from build123d import *

# Parameters (mm, degrees)
ESBO_O1_W                = 51.12
ESBO_O1_H                = 44.13
ESBO_O1_R                = 2
RESSALTO_EXTRUS_O1_DEPTH = 3


with BuildPart() as part:
    # Esboço1 → Ressalto-extrusão1 (new body)
    with BuildSketch(Plane(origin=(0, 0, 0), x_dir=(1, 0, 0), z_dir=(0, 1, 0))):
        with Locations((11.56, 12.065)):
            Rectangle(ESBO_O1_W, ESBO_O1_H)
        with Locations(Location((31.12, 12.065, 0), (0, 0, 270))):
            Circle(ESBO_O1_R, mode=Mode.SUBTRACT)
        with Locations(Location((-8, 12.065, 0), (0, 0, 270))):
            Circle(ESBO_O1_R, mode=Mode.SUBTRACT)
        with Locations(Location((11.56, 28.13, 0), (0, 0, 270))):
            Circle(ESBO_O1_R, mode=Mode.SUBTRACT)
        with Locations(Location((11.56, -4, 0), (0, 0, 270))):
            Circle(ESBO_O1_R, mode=Mode.SUBTRACT)
        Polygon((23.12, 24.13), (23.12, 18.13), (27.12, 18.13), (27.12, 6), (23.12, 6), (23.12, 0), (0, 0), (0, 6), (-4, 6), (-4, 18.13), (0, 18.13), (0, 24.13), align=None, mode=Mode.SUBTRACT)
    extrude(amount=RESSALTO_EXTRUS_O1_DEPTH)


solid = part.part
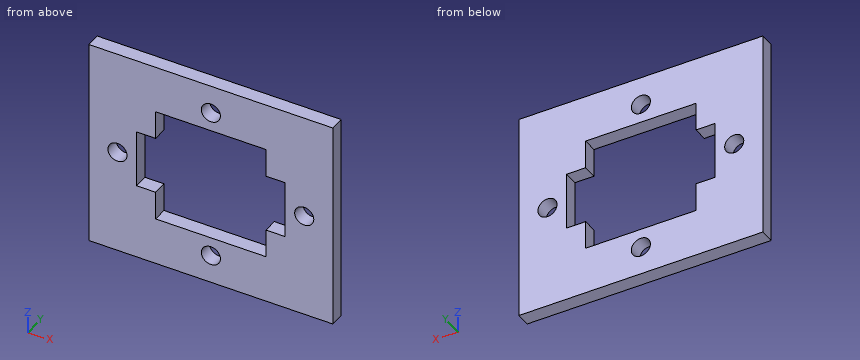
Here's how the part is built. I have some questions about the finished solid (model axes, mm). Coordinates: 2 decimals unless noted, no trailing zeros. Order: outer loops, then holes, each group sorted by start corner. A loop starts at its lowest first (then second) coordinate and runs counter-clockwise, first axis right, second up. Notation, with made-up numbers: (34.25, 29.25) -> (52.25, 29.25) arc R22 ccw to (52.25, 63.25) -> close; hole circle Ø11 at (-7, -2.5). An arc over 180 degrees is marked (long way). Answer in a Markdown table with one row per item.
(1) I want a section at D-D on x = 17.5. List the corners of the cut face in (y, z) for me, then the cut area to 3 significant figures.
Answer key:
| item | result |
|---|---|
| outline | (0, -34.13) -> (3, -34.13) -> (3, -24.13) -> (0, -24.13) -> close; (0, 0) -> (3, 0) -> (3, 10) -> (0, 10) -> close |
| area | 60.0 mm^2 |
(2) I want a section at B-B on z = 4. List the corners of the cut face in (x, y) for me, then the cut area to 3 significant figures.
Answer key:
| item | result |
|---|---|
| outline | (-14, 0) -> (9.56, 0) -> (9.56, 3) -> (-14, 3) -> close; (13.56, 0) -> (37.12, 0) -> (37.12, 3) -> (13.56, 3) -> close |
| area | 141 mm^2 |
(3) Will this pin go through, and if not, where does the flat tip stop? pin 1 Ø12 at (x, z) = (11.5, -23) entering from +Y.
Answer key:
| item | result |
|---|---|
| pin 1 | y = 3 |
(4) Please list where these lines run through material, in increasing order: probe 1 along Z at (x, y) = (25.5, 1.3); probe 2 along Z at (x, y) = (14.5, 0.8); probe 3 along X at (y, z) = (0.85, -18).
Answer key:
| item | result |
|---|---|
| probe 1 | -34.13 to -18.13, -6 to 10 |
| probe 2 | -34.13 to -24.13, 0 to 10 |
| probe 3 | -14 to -4, 27.12 to 37.12 |
(5) I want a section at A-A on x = 11.56. List the corners of the cut face in (y, z) for me, then the cut area to 3 significant figures.
Answer key:
| item | result |
|---|---|
| outline | (0, -34.13) -> (3, -34.13) -> (3, -30.13) -> (0, -30.13) -> close; (0, -26.13) -> (3, -26.13) -> (3, -24.13) -> (0, -24.13) -> close; (0, 0) -> (3, 0) -> (3, 2) -> (0, 2) -> close; (0, 6) -> (3, 6) -> (3, 10) -> (0, 10) -> close |
| area | 36.0 mm^2 |
(6) I want a section at C-C on y = 1.4. List the corners of the cut face in (x, z) for me (3 decimals).
Answer key:
| item | result |
|---|---|
| outline | (-14, -34.13) -> (37.12, -34.13) -> (37.12, 10) -> (-14, 10) -> close; hole circle Ø4 at (-8, -12.065); hole (-4, -18.13) -> (0, -18.13) -> (0, -24.13) -> (23.12, -24.13) -> (23.12, -18.13) -> (27.12, -18.13) -> (27.12, -6) -> (23.12, -6) -> (23.12, 0) -> (0, 0) -> (0, -6) -> (-4, -6) -> close; hole circle Ø4 at (11.56, -28.13); hole circle Ø4 at (11.56, 4); hole circle Ø4 at (31.12, -12.065) |
